Check sheet for the modelled part. Datum: model origin and axes. Units: mm. A direction names the side the tool comes from. Round coordinates to 2 decimals unless told otherwise and drop trailing zeros. Write each loop counter-clockwise with the first axis right and the second up, starting at its lowest first coordinate (ties: lowest second). Pieces come first, ordered by that corner, then holes. Notation, with made-up numbers: (-30.5, -35.5) -> (25.5, -35.5) arc R7 cw to (25.5, -31.5) -> close; hole circle Ø8 at (12, 46.5). An arc over 180 degrees is marked (long way). Use one line per item in the form item = value. Start each with the question number.
```python
from build123d import *

# Parameters (mm, degrees)
SKETCH1_W           = 44
SKETCH1_H           = 55.6
BOSS_EXTRUDE1_DEPTH = 3.175
SKETCH2_W           = 6.35
SKETCH2_H           = 41.5
SKETCH2_H_2         = 7.05
BOSS_EXTRUDE2_DEPTH = 20.6
BOSS_EXTRUDE3_DEPTH = 3.175
SKETCH5_R           = 2.25
CUT_EXTRUDE2_DEPTH  = 6.35
SKETCH6_R           = 1.65
CUT_EXTRUDE3_DEPTH  = 6.35
FILLET1_R           = 1
SKETCH7_W           = 6.35
SKETCH7_H           = 7.05
CUT_EXTRUDE4_DEPTH  = 3.175
FILLET2_R           = 1


with BuildPart() as part:
    # Sketch1 → Boss-Extrude1 (new body)
    with BuildSketch(Plane(origin=(0, 0, 0), x_dir=(1, 0, 0), z_dir=(0, 1, 0))):
        Rectangle(SKETCH1_W, SKETCH1_H)
    extrude(amount=BOSS_EXTRUDE1_DEPTH)

    # Sketch2 → Boss-Extrude2 (add)
    with BuildSketch(Plane(origin=(0, 3.175, 0), x_dir=(1, 0, 0), z_dir=(0, 1, 0))):
        with Locations((-18.825, 0)):
            Rectangle(SKETCH2_W, SKETCH2_H)
        with Locations((13.175, 24.275)):
            Rectangle(SKETCH2_W, SKETCH2_H_2)
        with Locations((13.175, -24.275)):
            Rectangle(SKETCH2_W, SKETCH2_H_2)
    extrude(amount=BOSS_EXTRUDE2_DEPTH)

    # Sketch3 → Boss-Extrude3 (add)
    with BuildSketch(Plane(origin=(0, 23.775, 0), x_dir=(1, 0, 0), z_dir=(0, 1, 0))):
        Polygon((-22, 20.75), (10, 20.75), (10, 27.8), (16.35, 27.8), (16.35, -27.8), (10, -27.8), (10, -20.75), (-22, -20.75), align=None)
    extrude(amount=BOSS_EXTRUDE3_DEPTH)

    # Sketch5 → Cut-Extrude2 (cut)
    with BuildSketch(Plane(origin=(16.35, 0, 0), x_dir=(0, 0, -1), z_dir=(1, 0, 0))):
        with Locations((-24.8, 8.425)):
            Circle(SKETCH5_R)
        with Locations((-24.8, 18.425)):
            Circle(SKETCH5_R)
        with Locations((24.8, 18.425)):
            Circle(SKETCH5_R)
        with Locations((24.8, 8.425)):
            Circle(SKETCH5_R)
    extrude(amount=-CUT_EXTRUDE2_DEPTH, mode=Mode.SUBTRACT)

    # Sketch6 → Cut-Extrude3 (cut)
    with BuildSketch(Plane.ZY.offset(22)):
        with Locations((10, 13.43)):
            Circle(SKETCH6_R)
    extrude(amount=-CUT_EXTRUDE3_DEPTH, mode=Mode.SUBTRACT)

    # Fillet1
    fillet1_edges = [part.edges().sort_by_distance(p)[0] for p in [
        (16.35, 13.475, 20.75),
        (16.35, 13.475, -20.75),
    ]]
    fillet(fillet1_edges, radius=FILLET1_R)

    # Sketch7 → Cut-Extrude4 (cut)
    with BuildSketch(Plane(origin=(0, 3.175, 0), x_dir=(1, 0, 0), z_dir=(0, 1, 0))):
        with Locations((-18.825, -24.275)):
            Rectangle(SKETCH7_W, SKETCH7_H)
        with Locations((-18.825, 24.275)):
            Rectangle(SKETCH7_W, SKETCH7_H)
    extrude(amount=-CUT_EXTRUDE4_DEPTH, mode=Mode.SUBTRACT)

    # Fillet2
    fillet2_edges = [part.edges().sort_by_distance(p)[0] for p in [
        (-15.65, 1.5875, 20.75),
        (-15.65, 1.5875, 27.8),
        (-15.65, 1.5875, -27.8),
        (-15.65, 1.5875, -20.75),
    ]]
    fillet(fillet2_edges, radius=FILLET2_R)


solid = part.part
```
1. Sectioned sample at C-C (y = 5.5). Enter the section's corners in (x, z).
2. Scan lines: probe 1 along Y at (x, z) = (13.5, 24.8) (3 decimals); probe 2 along Z at (x, y) = (15.5, 10); probe 3 along Y at (x, z) = (13, -18) (3 decimals). Record each from-to range of solid material in increasing order.
3. Tool access check on faces 4 (the face through (1, 23.775, 0)), 5 (the face through (2, 3.175, 0)), 6 (the face through (10, 15, 24)). Record the directions out of +Z, -Z, +X, -X, +Y, -Y that give a thin tool (end or side, any length) a straight path to the whole face; none if there is none.
4. Sectioned sample at D-D (z = -24.8). Enter the section's corners in (x, y) (3 decimals), and give its area (3 significant figures).
5. Sectioned sample at B-B (x = 5.5). Enter the section's corners in (y, z) (3 decimals), and give its area (3 significant figures).
6. Depth check by flat-ended pin: pin 1 (1 mm diameter, centred on y = 1.5, z = 25, fed in from -X); pin 2 (8 mm diameter, centred on x = -12, y = 17.5, fed in from -Z); pin 3 (4 mm diameter, centred on y = 20, z = -2, fed in from +X). Enter the tip coordinate at first touch or a pass-through.
7. Sectioned sample at A-A (z = 10). Enter the section's corners in (x, y) (3 decimals).
8. Mould release check, pull along Z, two halves, no side actions. Record for faces 1 (the face through (13, 13, -20.75)), 2 (the face through (11, 9, 27.8)), 3 (the face through (-15.65, 2, -24)): +Z half, -Z half, draft (parallel to the pull), parting line (faces both ways), or undercut.
Returned:
q1.outline = (-22, -20.75) -> (-15.65, -20.75) -> (-15.65, 20.75) -> (-22, 20.75) -> close; (10, -27.8) -> (16.35, -27.8) -> (16.35, -21.75) arc R1 ccw to (15.35, -20.75) -> (10, -20.75) -> close; (10, 20.75) -> (15.35, 20.75) arc R1 ccw to (16.35, 21.75) -> (16.35, 27.8) -> (10, 27.8) -> close
q2.probe_1 = 0 to 6.175, 10.675 to 16.175, 20.675 to 26.95
q2.probe_2 = -27.8 to -26.41, -23.19 to -20.76, 20.76 to 23.19, 26.41 to 27.8
q2.probe_3 = 0 to 3.175, 23.775 to 26.95
q3.face_4 = +X
q3.face_5 = none
q3.face_6 = +Z, -X, +Y
q4.outline = (-15.65, 0) -> (22, 0) -> (22, 3.175) -> (16.35, 3.175) -> (16.35, 6.175) -> (10, 6.175) -> (10, 3.175) -> (-15.65, 3.175) -> close; (10, 10.675) -> (16.35, 10.675) -> (16.35, 16.175) -> (10, 16.175) -> close; (10, 20.675) -> (16.35, 20.675) -> (16.35, 26.95) -> (10, 26.95) -> close
q4.area = 213 mm^2
q5.outline = (0, -27.8) -> (3.175, -27.8) -> (3.175, 27.8) -> (0, 27.8) -> close; (23.775, -20.75) -> (26.95, -20.75) -> (26.95, 20.75) -> (23.775, 20.75) -> close
q5.area = 308 mm^2
q6.pin_1 = -15.65
q6.pin_2 = -20.75
q6.pin_3 = -15.65
q7.outline = (-22, 0) -> (22, 0) -> (22, 3.175) -> (-15.65, 3.175) -> (-15.65, 11.78) -> (-22, 11.78) -> close; (-22, 15.08) -> (-15.65, 15.08) -> (-15.65, 23.775) -> (16.35, 23.775) -> (16.35, 26.95) -> (-22, 26.95) -> close
q8.face_1 = undercut
q8.face_2 = +Z half
q8.face_3 = draft
